Design review of the part built by this model. Coordinates are the model's own, in mm. Coordinates: 2 decimals unless noted, no trailing zeros. Write each loop counter-clockwise with the first axis right and the second up, starting at its lowest first coordinate (ties: lowest second). Pieces come first, ordered by that corner, then holes.
Autodesk Inventor part; units mm, degrees
ref_plane "body_right_vert_XY" through (0, 0, 0) normal (0, 0, -1) x (1, 0, 0)
ref_plane "body_right_vert_YZ" through (0, 0, 0) normal (1, 0, 0) x (0, -1, 0)
ref_plane "body_right_vert_ZX" through (0, 0, 0) normal (0, -1, 0) x (0, 0, -1)
sketch "Sketch_44" plane through (0, 0.254, 0) normal (0, 1, 0) x (1, 0, 0)
  line L0 (-1.27, -5.08) -> (1.27, -5.08)
  line L1 (1.27, -5.08) -> (1.27, 5.08)
  line L2 (1.27, 5.08) -> (-1.27, 5.08)
  line L3 (-1.27, 5.08) -> (-1.27, -5.08)
extrude "Extrusion1" add sketch "Sketch_44" along normal blind 0.0254
sketch "Sketch_2" plane through (0, 0, 0) normal (0, 0, 1) x (1, 0, 0)
  line L0 (-0.889, 0.254) -> (-0.889, -1.2192)
  line L1 (-0.889, -1.2192) -> (-0.5842, -1.2192)
  line L2 (-0.5842, -1.2192) -> (-0.5842, -5.4356)
  arc A0 (-0.5842, -5.4356) -> (0.5842, -5.4356) centre (0, -5.4356) ccw
  line L3 (0.5842, -5.4356) -> (0.5842, -1.2192)
  line L4 (0.5842, -1.2192) -> (0.889, -1.2192)
  line L5 (0.889, -1.2192) -> (0.889, 0.254)
  line L6 (0.889, 0.254) -> (-0.889, 0.254)
extrude "Extrusion2" add sketch "Sketch_2" along normal mid plane 0.7874
sketch "Sketch_3" plane through (0, 0, 4.699) normal (0, 0, 1) x (1, 0, 0)
  line L0 (-0.889, 0.254) -> (-0.889, -1.2192)
  line L1 (-0.889, -1.2192) -> (-0.5842, -1.2192)
  line L2 (-0.5842, -1.2192) -> (-0.5842, -5.4356)
  arc A0 (-0.5842, -5.4356) -> (0.5842, -5.4356) centre (0, -5.4356) ccw
  line L3 (0.5842, -5.4356) -> (0.5842, -1.2192)
  line L4 (0.5842, -1.2192) -> (0.889, -1.2192)
  line L5 (0.889, -1.2192) -> (0.889, 0.254)
  line L6 (0.889, 0.254) -> (-0.889, 0.254)
extrude "Extrusion3" add sketch "Sketch_3" along normal mid plane 0.7874
sketch "Sketch_4" plane through (0, 0, -4.699) normal (0, 0, 1) x (1, 0, 0)
  line L0 (-0.889, 0.254) -> (-0.889, -1.2192)
  line L1 (-0.889, -1.2192) -> (-0.5842, -1.2192)
  line L2 (-0.5842, -1.2192) -> (-0.5842, -5.4356)
  arc A0 (-0.5842, -5.4356) -> (0.5842, -5.4356) centre (0, -5.4356) ccw
  line L3 (0.5842, -5.4356) -> (0.5842, -1.2192)
  line L4 (0.5842, -1.2192) -> (0.889, -1.2192)
  line L5 (0.889, -1.2192) -> (0.889, 0.254)
  line L6 (0.889, 0.254) -> (-0.889, 0.254)
extrude "Extrusion4" add sketch "Sketch_4" along normal mid plane 0.7874
ref_plane "body_right_vert_XY" through (0, 0, 0) normal (0, 0, -1) x (1, 0, 0)
ref_plane "body_right_vert_YZ" through (0, 0, 0) normal (1, 0, 0) x (0, -1, 0)
ref_plane "body_right_vert_ZX" through (0, 0, 0) normal (0, -1, 0) x (0, 0, -1)
ref_plane "body_straight_XY" through (0, 0, 0) normal (0, -1, 0) x (1, 0, 0)
ref_plane "body_straight_YZ" through (0, 0, 0) normal (1, 0, 0) x (0, 0, 1)
ref_plane "body_straight_ZX" through (0, 0, 0) normal (0, 0, 1) x (0, -1, 0)
properties part number "M2T1SW03trmnls"
(1) Consider section D-D (y = -2.5). Give the boundary of the cut face in (x, z).
(2) Mouldability with a two-part tool opening along Z and no side actions: class faces 1 (the flat face through (0, -3, 5.093)), 2 (the flat face through (0, -3, -5.093)), 3 (the flat face through (0, 0.279, 0)), 4 (the flat face through (0, -3, -0.394)) as +Z half, -Z half, draft (parallel to the pull), parting line (faces both ways), or undercut.
(3) Consider section A-A (y = -0.25). Give the boundary of the cut face in (x, z).
(4) Wall thickness on line 1 (Z direction, x = 0.1, y = -4.75); line 2 (X direction, y = -5, z = -0.25); line 3 (X direction, y = -1, z = 0): over which ranges is each line inside the solid? List them lowest first.
(5) Insertion check: pin 1 Ø0.8 at (x, z) = (-0.5, 0.5) entering from -Y; pin 2 Ø0.6 at (y, z) = (-4, 4.5) entering from -X; pin 3 Ø2 at (y, z) = (-2, 0) entering from +X. Each pin has a flat end and moves straight along its axis. Give the tip position at first contact, or say it passes through.
Results:
1. outline: (-0.58, -5.09) - (0.58, -5.09) - (0.58, -4.31) - (-0.58, -4.31) - close; (-0.58, -0.39) - (0.58, -0.39) - (0.58, 0.39) - (-0.58, 0.39) - close; (-0.58, 4.31) - (0.58, 4.31) - (0.58, 5.09) - (-0.58, 5.09) - close
2. face 1: +Z half
2. face 2: -Z half
2. face 3: draft
2. face 4: undercut
3. outline: (-0.89, -5.09) - (0.89, -5.09) - (0.89, -4.31) - (-0.89, -4.31) - close; (-0.89, -0.39) - (0.89, -0.39) - (0.89, 0.39) - (-0.89, 0.39) - close; (-0.89, 4.31) - (0.89, 4.31) - (0.89, 5.09) - (-0.89, 5.09) - close
4. line 1: z = -5.09 to -4.31, -0.39 to 0.39, 4.31 to 5.09
4. line 2: x = -0.58 to 0.58
4. line 3: x = -0.89 to 0.89
5. pin 1: stops at y = -6.01
5. pin 2: stops at x = -0.58
5. pin 3: stops at x = 0.89
